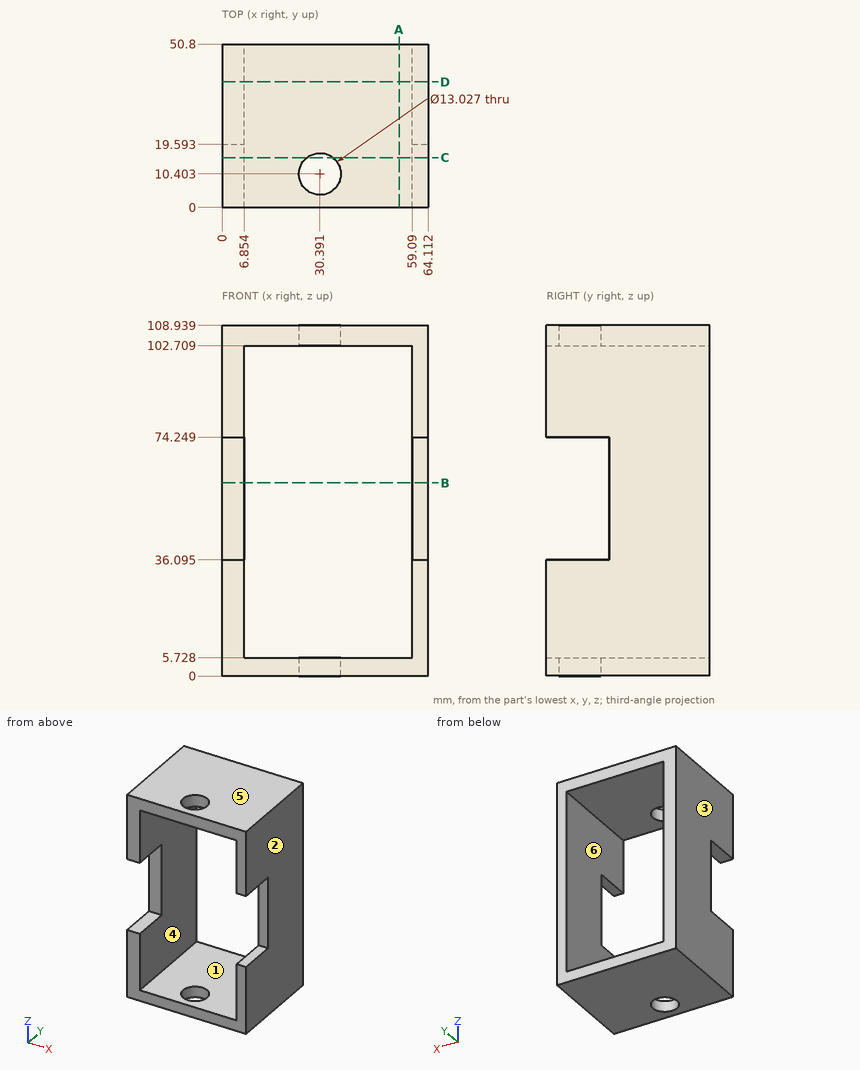
Study the drawing (mm; zero at the part's minimum x, y, z) and answer. A direction names the side the tool comes from. Coordinates: 2 decimals unless noted, no trailing zeros. Write each loop counter-clockwise with the first axis right and the second up, starting at its lowest first coordinate (ties: lowest second). Pieces come first, ordered by that corner, then holes. Notation, with made-up numbers: (43.5, 47) -> (92.5, 47) arc R23 cw to (92.5, 70) -> close; hole circle Ø11 at (-12, -39.75). An arc over 180 degrees is marked (long way). Write each question's results on one line, items separated by ' | '. Start each with the question number.
1) Flat-ended cylindrical pins translate along their axes: pin 1 Ø5.5 at (x, z) = (3.5, 58) entering from -Y; pin 2 Ø10 at (x, z) = (32, 94.5) entering from +Y; pin 3 Ø15 at (x, y) = (30.39, 10.4) entering from -Z. Find the tip coordinate at first contact, or state that the pin passes through.
2) Straight lines are drawn through the part: probe 1 along Z at (x, y) = (20.5, 40.5); probe 2 along X at (y, z) = (32, 49.5) (1 decimal); probe 3 along Y at (x, z) = (3, 67.5). For each, find the intervals that lie inside material, in ascending order.
3) A cutting plane is placed at A-A (x = 55). Determine the outline of the cut face in (y, z).
4) For a pull along X with two mould halves and no side action, classify the marked faces 3, 4, 5 and 6 as +X half, -X half, draft (parallel to the pull), parting line (faces both ways), or undercut.
5) A cutting plane is placed at C-C (y = 15.5). Determine the outline of the cut face in (x, z) (1 decimal), then the cut area to 3 significant figures.
6) A cutting plane is placed at B-B (z = 60). Determine the outline of the cut face in (x, y) (1 decimal).
7) A cutting plane is placed at D-D (y = 39). Determine the outline of the cut face in (x, z) (1 decimal).
8) A tool of negligible diameter and unlimited length cuts with its end or side. For the marked faces 1 and 2, from which of +Z, -Z, +X, -X, +Y, -Y can it reach the whole face along a straight path? Write none if from no direction.
Values follow:
1) pin 1: y = 19.59 | pin 2: through | pin 3: z = 0
2) probe 1: 0 to 5.73, 102.71 to 108.94 | probe 2: 0 to 6.9, 59.1 to 64.1 | probe 3: 19.59 to 50.8
3) outline: (0, 0) -> (50.8, 0) -> (50.8, 5.73) -> (0, 5.73) -> close; (0, 102.71) -> (50.8, 102.71) -> (50.8, 108.94) -> (0, 108.94) -> close
4) face 3: -X half | face 4: undercut | face 5: draft | face 6: undercut
5) outline: (0, 0) -> (26.3, 0) -> (26.3, 5.7) -> (6.9, 5.7) -> (6.9, 36.1) -> (0, 36.1) -> close; (0, 74.2) -> (6.9, 74.2) -> (6.9, 102.7) -> (26.3, 102.7) -> (26.3, 108.9) -> (0, 108.9) -> close; (34.4, 0) -> (64.1, 0) -> (64.1, 36.1) -> (59.1, 36.1) -> (59.1, 5.7) -> (34.4, 5.7) -> close; (34.4, 102.7) -> (59.1, 102.7) -> (59.1, 74.2) -> (64.1, 74.2) -> (64.1, 108.9) -> (34.4, 108.9) -> close | area: 1,370 mm²
6) outline: (0, 19.6) -> (6.9, 19.6) -> (6.9, 50.8) -> (0, 50.8) -> close; (59.1, 19.6) -> (64.1, 19.6) -> (64.1, 50.8) -> (59.1, 50.8) -> close
7) outline: (0, 0) -> (64.1, 0) -> (64.1, 108.9) -> (0, 108.9) -> close; hole (6.9, 5.7) -> (59.1, 5.7) -> (59.1, 102.7) -> (6.9, 102.7) -> close
8) face 1: +Y, -Y | face 2: +Z, -Z, +X, +Y, -Y
